Geometry: final body of the model. Coordinates: model frame, mm. A direction names the side the tool comes from. Give positions to 0.01 mm unless a question says otherwise; leave off trailing zeros. Order: outer loops, then holes, each group sorted by start corner. A loop starts at its lowest first (then second) coordinate and runs counter-clockwise, first axis right, second up. Notation, with made-up numbers: (-18.75, -21) - (25.25, -21) arc R11 ccw to (25.25, -7) - close; hole circle Ø10 at (-36.5, -17). An arc over 180 degrees is marked (long way). One line per item, written item: value.
```python
from build123d import *

# Parameters (mm, degrees)
BOSS_EXTRUDE1_DEPTH = 2.5
CUT_EXTRUDE1_DEPTH  = 8
CIRPATTERN1_COUNT   = 14
CUT_EXTRUDE2_START  = -10
SKETCH5_R           = 5
CUT_EXTRUDE2_DEPTH  = 10


with BuildPart() as part:
    # Sketch1 → Revolve1 (revolve)
    with BuildSketch(Plane.XY, mode=Mode.PRIVATE) as revolve1_sk:
        Polygon((-5, -1.7), (-5, -14.966593737), (-7, -14.966593737), (-8.41, -14.152529857), (-7, -13.338465977), (-8.41, -12.524402098), (-7, -11.710338218), (-8.41, -10.896274339), (-7, -10.082210459), (-8.41, -9.26814658), (-7, -8.4540827), (-8.41, -7.640018821), (-7, -7), (-7, -2), (-8.481548045, -1.144627838), (-7, -0.289255675), (-8.481548045, 0.566116487), (-7, 1.42148865), (-8.481548045, 2.276860812), (-7, 3.132232974), (-8.481548045, 3.987605137), (-7, 4.842977299), (-8.481548045, 5.698349462), (-7, 6.553721624), (-6.800767408, 6.553721624), (-6.577224477, 6.553721624), (-6.577224477, 7), (-7, 7), (-7, 15), (-5.371576334, 15), (-5.753711326, 7), (-5.371576334, 7), (-4.595145819, 7), align=None)
    revolve(revolve1_sk.sketch.rotate(Axis((0, -16.464923423, 0), (0, 1, 0)), 270), axis=Axis((0, -16.464923423, 0), (0, 1, 0)))

    # Sketch2 → Boss-Extrude1 (add, symmetric)
    with BuildSketch(Plane.XZ.offset(4.466593737)):
        Polygon((10.969655115, 0), (5.484827557, 9.5), (-5.484827557, 9.5), (-10.969655115, 0), (-5.484827557, -9.5), (5.484827557, -9.5), align=None)
    extrude(amount=BOSS_EXTRUDE1_DEPTH, both=True)

    # Sketch4 → Cut-Extrude1 (cut)
    with BuildSketch(Plane(origin=(0, 15, 0), x_dir=(1, 0, 0), z_dir=(0, 1, 0))):
        Polygon((-8.353753696, 8.845150972), (-2.200605193, 0.256381188), (-2.627907173, 0), (-8.80128537, 8.617007067), align=None)
    cut_extrude1 = extrude(amount=-CUT_EXTRUDE1_DEPTH, mode=Mode.SUBTRACT)

    # CirPattern1: Cut-Extrude1 ×14 about axis
    cirpattern1_axis = Axis((0, 0, 0), (0, 1, 0))
    for i in range(1, CIRPATTERN1_COUNT):
        add(cut_extrude1.rotate(cirpattern1_axis, i * 360 / CIRPATTERN1_COUNT), mode=Mode.SUBTRACT)

    # Sketch5 → Cut-Extrude2 (cut)
    with BuildSketch(Plane(origin=(0, -1.966593737, 0), x_dir=(1, 0, 0), z_dir=(0, 1, 0)).offset(CUT_EXTRUDE2_START)):
        with Locations(Location((0, 0, 0), (0, 0, 90))):
            Circle(SKETCH5_R)
    extrude(amount=CUT_EXTRUDE2_DEPTH, mode=Mode.SUBTRACT)


solid = part.part
```
1) Section A-A, the plane y = -2.5. Return loops of the section in (x, z).
Answers below:
outline: (-10.97, 0) - (-5.48, -9.5) - (5.48, -9.5) - (10.97, 0) - (5.48, 9.5) - (-5.48, 9.5) - close; hole circle Ø10 at (0, 0)
2) Set-up query: faces 1 (the face through (6.29, 11.06, 3.07)), 2 (the face through (-2.732, 11.056, 5.558)), 3 (the face through (6.42, 6.78, 1.43)). Return all of +Z, -Z, +X, -X, +Y, -Y with unobstructed straight access to the full face (end or side cutting, diameter ignored); none if empty.
Answers below:
face 1: +Z, +X, +Y
face 2: +Y
face 3: none
3) Material intervals for line 1 along Y through (x, z) = (-6.75, 5.5); line 2 along Y through (x, z) = (-5, -1.75); line 3 along X through (y, z) = (-13.5, -1.5), sorted ascending.
Answers below:
line 1: -6.97 to -1.97
line 2: -14.97 to 7
line 3: -7.12 to -4.77, 4.77 to 7.12
4) First-contact query: pin 1 (10.5 mm diameter, centred on x = 2, z = -1.5, fed in from +Y); pin 2 (2 mm diameter, centred on y = -4, z = 4, fed in from +X); pin 3 (1.5 mm diameter, centred on y = -8.5, z = 3, fed in from -X); pin 4 (1.5 mm diameter, centred on y = -2.5, z = 4.5, fed in from +X). Flat tips, straight axial feed; report the tip coordinate or a pass-through.
Answers below:
pin 1: y = 15
pin 2: x = 9.24
pin 3: x = -7.85
pin 4: x = 8.8
5) Section B-B, the plane y = 5.25. Return loops of the section in (x, z).
Answers below:
outline: circle Ø15.41 at (0, 0); hole circle Ø9.35 at (0, 0)
6) Mould query, pull axis X, two halves, no side actions, for faces 4 (the face through (1.522, 11.056, 6.833)), 5 (the face through (0.05, 11.06, -6.19)), 6 (the face through (-4.87, 11.06, 3.82)), 7 (the face through (-4, 15, 5)). Classes: released by +X, released by -X, zero draft, split by the parting line, or undercut.
Answers below:
face 4: released by +X
face 5: undercut
face 6: undercut
face 7: zero draft
